from build123d import *

# Parameters (mm, degrees)
F1_DEPTH = 5
F3_DEPTH = 75
F5_DEPTH = 58.501
F7_DEPTH = 5.001
F8_R     = 1
F9_DEPTH = 67.142736129


with BuildPart() as f1:
    # F0 (on Top) → F1 (new body)
    with BuildSketch(Plane.XY):
        with BuildLine():
            ThreePointArc((37.148351242, -24.5), (0, 44.5), (-37.148351242, -24.5))
            Line((-37.148351242, -24.5), (37.148351242, -24.5))
        make_face()
    extrude(amount=F1_DEPTH)

    # F2 (on face) → F3 (join)
    with BuildSketch(Plane.XY.offset(5)):
        with BuildLine():
            Line((-14, -24.5), (0, -24.5))
            Line((0, -24.5), (14, -24.5))
            Line((14, -24.5), (14, 42.240383521))
            ThreePointArc((14, 42.240383521), (0, 44.5), (-14, 42.240383521))
            Line((-14, 42.240383521), (-14, -24.5))
        make_face()
    extrude(amount=F3_DEPTH)

    # F4 (on face) → F5 (cut, through all)
    with BuildSketch(Plane.YZ.offset(14)):
        Polygon((-24.5, 5), (0, 80), (0, 88), (-35, 88), (-35, 5), align=None)
        Polygon((57.2117942726, 88), (32.2117942726, 88), (32.2117942726, 80), (44.5, 5), (57.2117942726, 5), align=None)
    extrude(amount=-F5_DEPTH, mode=Mode.SUBTRACT)

    # F6 (on face) → F7 (cut, through all)
    with BuildSketch(Plane.XY.offset(5)):
        Polygon((-33.5, -2.5), (-33.5, 0), (-33.5, 2.5), (-35.5, 2.5), (-35.5, -2.5), align=None)
        Polygon((35.5, 2.5), (33.5, 2.5), (33.5, 0), (33.5, -2.5), (35.5, -2.5), align=None)
    extrude(amount=-F7_DEPTH, mode=Mode.SUBTRACT)

    # F8 (on face) → F9 (cut, through all)
    with BuildSketch(Plane(origin=(0, -23.6135094976, 7.7137464359), x_dir=(1, 0, 0), z_dir=(0, -0.9505672883, 0.3105186475))):
        with Locations((0, 76.0453830625)):
            Circle(F8_R)
        with Locations((-4, 76.0453830625)):
            Circle(F8_R)
    extrude(amount=-F9_DEPTH, mode=Mode.SUBTRACT)


solid = f1.part
The model under review builds one solid part; all positions refer to its coordinate system, in mm. A direction names the side the tool comes from. Round coordinates to 2 decimals unless told otherwise and drop trailing zeros. Order: outer loops, then holes, each group sorted by start corner. A loop starts at its lowest first (then second) coordinate and runs counter-clockwise, first axis right, second up. Notation, with made-up numbers: (21.5, -16.75) -> (64.5, -16.75) arc R17 cw to (64.5, 1.25) -> close; hole circle Ø3 at (-16.5, 81.5). An arc over 180 degrees is marked (long way). Use CSV: the item, a comma, the result in double quotes. Start each with the question number.
(1) Mouldability with a two-part tool opening along Z and no side actions: class faces 6 (the face through (-26, 2, 5)), 7 (the face through (-1, 10, 0)), 8 (the face through (33.5, 0, 3)), 9 (the face through (0.5, 16.8, 73.6)) as pulls with the +Z half, pulls with the -Z half, needs draft (parallel to the pull), parting line crosses it, or undercut.
(2) Consider section D-D on y = 16. State how many separate pieces and enclosed holes the cut face has, and give its area (3 significant figures).
(3) Wall thickness on probe 1 along Z at (x, y) = (-15, 32); probe 2 along X at (y, z) = (24, 21.5); probe 3 along Y at (x, z) = (-6, 49): over which ranges is each line inside the solid? List them lowest first. Write a range as from..to.
(4) Consider section B-B on y = 37. Write out the cut boundary in (x, z).
(5) Consider section A-A on x = 11. Write out the cut boundary in (y, z).
(6) Consider section C-C on z = 9. Write out the cut boundary in (x, y).
(7) Tool access review of faces 1 (the face through (-33.5, 0, 3)), 2 (the face through (-14, 9, 34)), 3 (the face through (14, 16, 42)), 4 (the face through (0, 16, 80)), 5 (the face through (0.2, -12.42, 41.98)): name each direction out of +Z, -Z, +X, -X, +Y, -Y from which nothing blocks a thin tool from reaching the whole face with its end or side.
(8) Insertion check: pin 1 (8 mm diameter, centred on x = 30, y = 32.5, fed in from +Z); pin 2 (5.5 mm diameter, centred on y = 1, z = 3.5, fed in from +X); pin 3 (1.5 mm diameter, centred on y = -14.5, z = 9, fed in from +X); pin 4 (5 mm diameter, centred on x = 11, z = 30.5, fed in from -Y). Each pin has a flat end and moves straight along its axis. Give the tip position at first contact, or say it passes through.
Responses:
1,face 6,"pulls with the +Z half"
1,face 7,"pulls with the -Z half"
1,face 8,"needs draft"
1,face 9,"undercut"
2,separate pieces,"1"
2,enclosed holes,"2"
2,area,"2,510 mm²"
3,probe 1,"0..5"
3,probe 2,"-14..14"
3,probe 3,"-10.13..37.29"
4,outline,"(-24.72, 0) -> (24.72, 0) -> (24.72, 5) -> (14, 5) -> (14, 50.78) -> (-14, 50.78) -> (-14, 5) -> (-24.72, 5) -> close"
5,outline,"(-24.5, 0) -> (43.12, 0) -> (43.12, 13.43) -> (32.21, 80) -> (0, 80) -> (-24.5, 5) -> close"
6,outline,"(-14, -23.19) -> (14, -23.19) -> (14, 42.24) arc R44.5 ccw to (7.61, 43.84) -> (-7.61, 43.84) arc R44.5 ccw to (-14, 42.24) -> close"
7,face 1,"+Z, -Z"
7,face 2,"+Z, -X, +Y, -Y"
7,face 3,"+Z, +X, +Y, -Y"
7,face 4,"+Z, +X, -X, +Y, -Y"
7,face 5,"+Z, +X, -X, -Y"
8,pin 1,"z = 5"
8,pin 2,"x = 44.5"
8,pin 3,"x = 14"
8,pin 4,"y = -16.99"
